Geometry: final body of the model. Coordinates: model frame, mm. Face numbers are marked on the shaded views. Coordinates: 2 decimals unless noted, no trailing zeros. Write each loop counter-clockwise with the first axis right and the second up, starting at its lowest first coordinate (ties: lowest second). Pieces come first, ordered by that corner, then holes. Notation, with made-up numbers: (-31.5, 73.5) -> (-5.5, 73.5) arc R15 ccw to (-5.5, 77.5) -> close; hole circle Ø4 at (40, 8). An arc over 180 degrees is marked (long way). Answer as a JSON object with one key per item and string values. Group by question number.
```python
from build123d import *

# Parameters (mm, degrees)
F0_W     = 460
F0_H     = 738
F1_DEPTH = 1.5
F2_W     = 460
F2_H     = 738
F2_W_2   = 457
F2_H_2   = 735
F3_DEPTH = 25
F4_R     = 4
F5_DEPTH = 25
F6_R     = 4
F7_DEPTH = 25


with BuildPart() as f1:
    # F0 (on Top) → F1 (new body)
    with BuildSketch(Plane.XY):
        Rectangle(F0_W, F0_H)
        with BuildLine():
            Line((-100, 219), (100, 219))
            ThreePointArc((100, 219), (121.213203, 210.213203), (130, 189))
            Line((130, 189), (130, -189))
            ThreePointArc((130, -189), (121.213203, -210.213203), (100, -219))
            Line((100, -219), (-100, -219))
            ThreePointArc((-100, -219), (-121.213203, -210.213203), (-130, -189))
            Line((-130, -189), (-130, 189))
            ThreePointArc((-130, 189), (-121.213203, 210.213203), (-100, 219))
        make_face(mode=Mode.SUBTRACT)
    extrude(amount=F1_DEPTH)

    # F2 (on face) → F3 (join)
    with BuildSketch(Plane.XY.offset(1.5)):
        Rectangle(F2_W, F2_H)
        Rectangle(F2_W_2, F2_H_2, mode=Mode.SUBTRACT)
    extrude(amount=F3_DEPTH)

    # F4 (on face) → F5 (cut)
    with BuildSketch(Plane.YZ.offset(230)):
        with Locations((-69, 16.5)):
            Circle(F4_R)
        with Locations((331, 16.5)):
            Circle(F4_R)
    extrude(amount=-F5_DEPTH, mode=Mode.SUBTRACT)

    # F6 (on face) → F7 (cut)
    with BuildSketch(Plane(origin=(-230, 0, 0), x_dir=(0, -1, 0), z_dir=(-1, 0, 0))):
        with Locations((-331, 16.5)):
            Circle(F6_R)
        with Locations((69, 16.5)):
            Circle(F6_R)
    extrude(amount=-F7_DEPTH, mode=Mode.SUBTRACT)


solid = f1.part
```
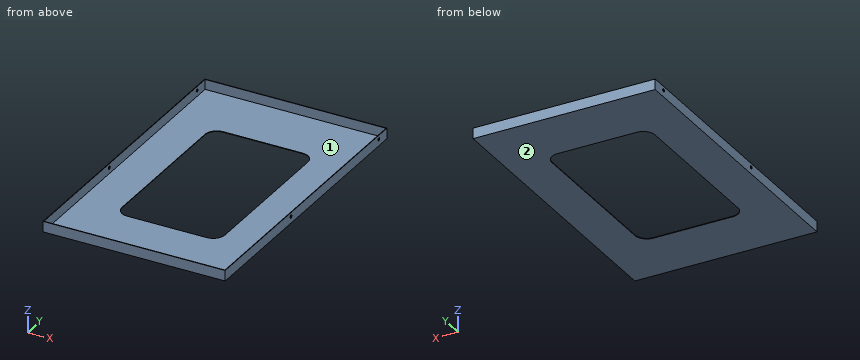
Item 1: Section C-C on y = -278.5. Output: boundary loops of the cut face in (x, z).
Item 2: Mould query, pull axis Y, two halves, no side actions, for the marked faces 1 and 2. Classes: +Y half, -Y half, draft (parallel to the pull), parting line (faces both ways), or undercut.
Item 3: Section B-B on z = 16.5. Output: boundary loops of the cut face in (x, y), then the cut area to 3 significant figures.
Item 4: Section A-A on x = -14. Output: boundary loops of the cut face in (y, z).
Item 5: Ray query, L1, parallel to X at y = -249.5, z = 11.5; L2, parallel to Y at x = -42.5, z = 23; L3, parallel to Z at x = -229.7, y = 331. Return the intervals inside material, ascending. Write a range as [from, to].
Item 6: Section D-D on y = 208.5. Output: boundary loops of the cut face in (x, z).
Item 7: Contact query for flat-ended pins moving along their axis: pin 1 (9 mm diameter, centred on y = -69, z = 16.5, fed in from +X); pin 2 (12 mm diameter, centred on x = -149.5, y = 251, fed in from +Z). Output: stop coordinate, or through.
Answer sheet:
{
 "1": {"outline": "(-230, 0) -> (230, 0) -> (230, 26.5) -> (228.5, 26.5) -> (228.5, 1.5) -> (-228.5, 1.5) -> (-228.5, 26.5) -> (-230, 26.5) -> close"},
 "2": {"face 1": "undercut", "face 2": "draft"},
 "3": {"outline": "(-230, -369) -> (230, -369) -> (230, -73) -> (228.5, -73) -> (228.5, -367.5) -> (-228.5, -367.5) -> (-228.5, -73) -> (-230, -73) -> close; (-230, -65) -> (-228.5, -65) -> (-228.5, 327) -> (-230, 327) -> close; (-230, 335) -> (-228.5, 335) -> (-228.5, 367.5) -> (228.5, 367.5) -> (228.5, 335) -> (230, 335) -> (230, 369) -> (-230, 369) -> close; (228.5, -65) -> (230, -65) -> (230, 327) -> (228.5, 327) -> close", "area": "3,540 mm^2"},
 "4": {"outline": "(-369, 0) -> (-219, 0) -> (-219, 1.5) -> (-367.5, 1.5) -> (-367.5, 26.5) -> (-369, 26.5) -> close; (219, 0) -> (369, 0) -> (369, 26.5) -> (367.5, 26.5) -> (367.5, 1.5) -> (219, 1.5) -> close"},
 "5": {"L1": "x = [-230, -228.5], [228.5, 230]", "L2": "y = [-369, -367.5], [367.5, 369]", "L3": "z = [0, 12.5], [20.5, 26.5]"},
 "6": {"outline": "(-230, 0) -> (-122.8, 0) -> (-122.8, 1.5) -> (-228.5, 1.5) -> (-228.5, 26.5) -> (-230, 26.5) -> close; (122.8, 0) -> (230, 0) -> (230, 26.5) -> (228.5, 26.5) -> (228.5, 1.5) -> (122.8, 1.5) -> close"},
 "7": {"pin 1": "stops at x = 230", "pin 2": "stops at z = 1.5"}
}
